```python
from build123d import *

# Parameters (mm, degrees)
F0_W     = 60
F0_H     = 13
F1_DEPTH = 5
F3_D     = 3
F4_W     = 60
F4_H     = 3
F5_DEPTH = 28
F6_W     = 25
F6_H     = 25
F7_DEPTH = 5
F9_D     = 2
F10_R    = 15


with BuildPart() as f1:
    # F0 (on Top) → F1 (new body)
    with BuildSketch(Plane.XY):
        with Locations((30, 6.5)):
            Rectangle(F0_W, F0_H)
    extrude(amount=F1_DEPTH)

    # F3 (through all)
    with Locations(Plane.XY.offset(5)):
        with Locations((5, 5), (55, 5)):
            Hole(F3_D / 2)

    # F4 (on face) → F5 (join)
    with BuildSketch(Plane.XY.offset(5)):
        with Locations((30, 11.5)):
            Rectangle(F4_W, F4_H)
    extrude(amount=F5_DEPTH)

    # F6 (on face) → F7 (cut)
    with BuildSketch(Plane(origin=(0, 13, 0), x_dir=(-1, 0, 0), z_dir=(0, 1, 0))):
        with Locations((-30, 20.5)):
            Rectangle(F6_W, F6_H)
    extrude(amount=-F7_DEPTH, mode=Mode.SUBTRACT)

    # F9 (through all)
    with Locations(Plane(origin=(0, 13, 0), x_dir=(-1, 0, 0), z_dir=(0, 1, 0))):
        with Locations((-44, 30.5), (-16, 10.5)):
            Hole(F9_D / 2)

    # F10
    f10_edges = [f1.edges().sort_by_distance(p)[0] for p in [
        (0, 11.5, 33),
        (60, 11.5, 33),
    ]]
    fillet(f10_edges, radius=F10_R)


solid = f1.part
```
The model under review builds one solid part; all positions refer to its coordinate system, in mm. A direction names the side the tool comes from. Give positions to 0.01 mm unless a question says otherwise; leave off trailing zeros. Write each loop counter-clockwise with the first axis right and the second up, starting at its lowest first coordinate (ties: lowest second). Pieces come first, ordered by that corner, then holes. Notation, with made-up numbers: (41.5, -22) - (54.5, -22) arc R16 ccw to (54.5, 9) - close; hole circle Ø3 at (51.5, 60). An arc over 180 degrees is marked (long way). Answer in a Markdown table with one row per item. Add a question column.
1. Wall thickness on line 1 along Y through (x, z) = (5, 1.35); line 2 along Z through (x, y) = (16, 10.7); line 3 along X through (y, z) = (12, 13.5): over which ranges is each line inside the solid? List them lowest first. Write a range as [from, to].
2. We need section A-A on z = 10.5. Write out the cut boundary in (x, y).
3. Tool access review of faces 1 (the cylindrical face through (6.2, 4.1, 2.5)), 2 (the flat face through (42.5, 12, 20)), 3 (the flat face through (30, 10, 6)): name each direction out of +Z, -Z, +X, -X, +Y, -Y from which nothing blocks a thin tool from reaching the whole face with its end or side.
4. We need section B-B on y = 5. Write out the cut boundary in (x, z).
5. We need section D-D on z = 21. Write out the cut boundary in (x, y), then the cut area to 3 significant figures.
6. We need section C-C on x = 5. Write out the cut boundary in (y, z), then the cut area to 3 significant figures.
7. Draft analysis for pull direction Z (two halves, no side actions). For faces 4 (the flat face through (30, 12, 8)), 5 (the cylindrical face through (16.954, 11.479, 10.8)), 6 (the cylindrical face through (44.954, 11.479, 30.8)), 7 (the flat face through (30, 7, 0)), state which applies: +Z half, -Z half, draft (parallel to the pull), parting line (faces both ways), or undercut.
8. Insertion check: P1, Ø3.5, axis at x = 33.5, y = 11, coming from the +Z side; P2, Ø1.5, axis at x = 47, z = 16.5, coming from the -Y side; P3, Ø0.9, axis at y = 11, z = 25.5, coming from the -X side. Each pin has a flat end and moves straight along its axis. Give the tip position at first contact, or say it passes through.
Ans:
| question | item | result |
|---|---|---|
| 1 | line 1 | y = [0, 3.5], [6.5, 13] |
| 1 | line 2 | z = [0, 9.5], [11.5, 33] |
| 1 | line 3 | x = [0, 17.5], [42.5, 60] |
| 2 | outline | (0, 10) - (15, 10) - (15, 13) - (0, 13) - close; (17, 10) - (17.5, 10) - (17.5, 13) - (17, 13) - close; (42.5, 10) - (60, 10) - (60, 13) - (42.5, 13) - close |
| 3 | face 1 | +Z, -Z |
| 3 | face 2 | +Z, +Y, -Y |
| 3 | face 3 | +Z, +X, -X, -Y |
| 4 | outline | (0, 0) - (3.5, 0) - (3.5, 5) - (0, 5) - close; (6.5, 0) - (53.5, 0) - (53.5, 5) - (6.5, 5) - close; (56.5, 0) - (60, 0) - (60, 5) - (56.5, 5) - close |
| 5 | outline | (0.3, 10) - (17.5, 10) - (17.5, 13) - (0.3, 13) - close; (42.5, 10) - (59.7, 10) - (59.7, 13) - (42.5, 13) - close |
| 5 | area | 103 mm^2 |
| 6 | outline | (0, 0) - (3.5, 0) - (3.5, 5) - (0, 5) - close; (6.5, 0) - (13, 0) - (13, 29.18) - (10, 29.18) - (10, 5) - (6.5, 5) - close |
| 6 | area | 123 mm^2 |
| 7 | face 4 | +Z half |
| 7 | face 5 | undercut |
| 7 | face 6 | undercut |
| 7 | face 7 | -Z half |
| 8 | P1 | stops at z = 8 |
| 8 | P2 | stops at y = 10 |
| 8 | P3 | stops at x = 1.76 |
